from build123d import *

# Parameters (mm, degrees)
SKETCH1_W           = 12
SKETCH1_H           = 20
BOSS_EXTRUDE1_DEPTH = 2
SKETCH2_W           = 2.583613584
SKETCH2_H           = 9.909750732
BOSS_EXTRUDE2_DEPTH = 3
SKETCH3_W           = 12
SKETCH3_H           = 20
BOSS_EXTRUDE3_DEPTH = 3
FILLET1_R           = 0.5


with BuildPart() as part:
    # Sketch1 → Boss-Extrude1 (new body)
    with BuildSketch(Plane.XY):
        with Locations((68.585871194, -163)):
            Rectangle(SKETCH1_W, SKETCH1_H)
    extrude(amount=BOSS_EXTRUDE1_DEPTH)

    # Sketch2 → Boss-Extrude2 (add)
    with BuildSketch(Plane.XY.offset(2)):
        with Locations((72.404631484, -158.933321579)):
            Rectangle(SKETCH2_W, SKETCH2_H)
    extrude(amount=BOSS_EXTRUDE2_DEPTH)

    # Sketch3 → Boss-Extrude3 (add)
    with BuildSketch(Plane.XY.offset(5)):
        with Locations((68.585871194, -163)):
            Rectangle(SKETCH3_W, SKETCH3_H)
    extrude(amount=BOSS_EXTRUDE3_DEPTH)

    # Fillet1
    fillet1_edges = [part.edges().sort_by_distance(p)[0] for p in [
        (62.585871194, -173, 6.5),
        (74.585871194, -173, 6.5),
        (74.585871194, -153, 6.5),
        (62.585871194, -153, 6.5),
        (62.585871194, -153, 1),
        (74.585871194, -153, 1),
        (74.585871194, -173, 1),
        (62.585871194, -173, 1),
    ]]
    fillet(fillet1_edges, radius=FILLET1_R)


solid = part.part
Design review of the part built by this model. Coordinates are the model's own, in mm. A direction names the side the tool comes from. Coordinates: 2 decimals unless noted, no trailing zeros. Loops run counter-clockwise (first coordinate to the right, second up) from the corner with the lowest first, then second, coordinate; pieces in that order, holes last. Notation, with made-up numbers: M 55,64 L 109,64 A15 cw 109,75 Z; hole C -9,69 d6. An arc over 180 degrees is marked long. Answer as CSV lines item,"result".
Item 1: Add section D-D on y = -157.75. State the section outline as (x, z) points.
Answer list:
outline,"M 62.59,0 L 74.59,0 L 74.59,2 L 73.7,2 L 73.7,5 L 74.59,5 L 74.59,8 L 62.59,8 L 62.59,5 L 71.11,5 L 71.11,2 L 62.59,2 Z"
Item 2: Machinability: for faces 1 (the face through (73.696, -159, 3)), 2 (the face through (71.113, -159, 3)), 3 (the face through (72, -163.888, 3)), which of the approach directions +Z, -Z, +X, -X, +Y, -Y give a long, thin tool a straight path to every point of the face, cutting with its end or side? Answer none if there is none.
Answer list:
face 1,"+X, +Y, -Y"
face 2,"-X, +Y, -Y"
face 3,"+X, -X, -Y"
Item 3: For probe 1 along Z at (x, y) = (66.5, -164); probe 2 along X at (y, z) = (-154.25, 2.25), list the stretches that pass through material, from the lowest coordinate up.
Answer list:
probe 1,"0 to 2, 5 to 8"
probe 2,"71.11 to 73.7"
Item 4: Add section A-A on x = 69. State the section outline as (y, z) points.
Answer list:
outline,"M -173,0 L -153,0 L -153,2 L -173,2 Z; M -173,5 L -153,5 L -153,8 L -173,8 Z"
Item 5: Add section C-C on x = 72.5. State the section outline as (y, z) points.
Answer list:
outline,"M -173,0 L -153,0 L -153,2 L -153.98,2 L -153.98,5 L -153,5 L -153,8 L -173,8 L -173,5 L -163.89,5 L -163.89,2 L -173,2 Z"
Item 6: For P1, Ø0.9, axis at y = -158, z = 3.5, coming from the -X side; P2, Ø0.8, axis at x = 72, z = 3.5, coming from the -Y side; P3, Ø1.5, axis at y = -159, z = 4, coming from the +X side, all flat-tipped, find the tip position at first contact; note any pin that passes through.
Answer list:
P1,"x = 71.11"
P2,"y = -163.89"
P3,"x = 73.7"
Item 7: Add section B-B on y = -167. State the section outline as (x, z) points.
Answer list:
outline,"M 62.59,0 L 74.59,0 L 74.59,2 L 62.59,2 Z; M 62.59,5 L 74.59,5 L 74.59,8 L 62.59,8 Z"
